Source: CAD feature listing. Evaluate the final solid. Frame: model axes, mm. Face numbers are marked on the shaded views. Round coordinates to 2 decimals unless told otherwise and drop trailing zeros. Write each loop counter-clockwise with the first axis right and the second up, starting at its lowest first coordinate (ties: lowest second). Pieces come first, ordered by that corner, then holes. Notation, with made-up numbers: M 57,-8 L 97,-8 A24 cw 97,5 Z; hole C 50,36 d6. An arc over 180 degrees is marked long. Use a Markdown table: item, result.
```python
from build123d import *

# Parameters (mm, degrees)
BOSS_EXTRUDE1_DEPTH = 10
SKETCH2_R           = 20.5
CUT_EXTRUDE1_DEPTH  = 5
SKETCH4_R           = 5
CUT_EXTRUDE3_DEPTH  = 166.604951617
SKETCH5_R           = 5
CUT_EXTRUDE4_DEPTH  = 5


with BuildPart() as part:
    # Sketch1 → Boss-Extrude1 (new body)
    with BuildSketch(Plane(origin=(0, 0, 0), x_dir=(0, 0, -1), z_dir=(1, 0, 0))):
        Polygon((-95, 70), (-140, 70), (-140, 55), (-150, 55), (-150, 15), (-140, 15), (-140, 0), (-95, 0), (-95, 5), (-55, 5), (-55, 0), (-10, 0), (-10, 15), (0, 15), (0, 55), (-10, 55), (-10, 70), (-55, 70), (-55, 60), (-95, 60), align=None)
    extrude(amount=BOSS_EXTRUDE1_DEPTH)

    # Sketch2 → Cut-Extrude1 (cut)
    with BuildSketch(Plane(origin=(10, 0, 0), x_dir=(0, 0, -1), z_dir=(1, 0, 0))):
        with Locations((-108.52, 40)):
            Circle(SKETCH2_R)
    extrude(amount=-CUT_EXTRUDE1_DEPTH, mode=Mode.SUBTRACT)

    # Sketch4 → Cut-Extrude3 (cut, through all)
    with BuildSketch(Plane(origin=(5, 0, 0), x_dir=(0, 0, -1), z_dir=(1, 0, 0))):
        with Locations((-108.52, 40)):
            Circle(SKETCH4_R)
    extrude(amount=-CUT_EXTRUDE3_DEPTH, mode=Mode.SUBTRACT)

    # Sketch5 → Cut-Extrude4 (cut)
    with BuildSketch(Plane.ZY):
        with Locations((37.080096083, 26.674400393)):
            Circle(SKETCH5_R)
        with Locations((72.52, 33)):
            Circle(SKETCH5_R)
    extrude(amount=-CUT_EXTRUDE4_DEPTH, mode=Mode.SUBTRACT)


solid = part.part
```
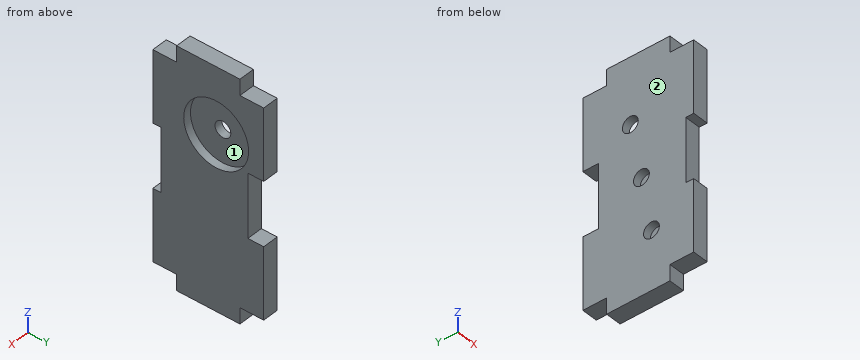
Q1. Section D-D on y = 40. Return loops of the section in (x, z).
Results are:
| item | result |
|---|---|
| outline | M 0,0 L 10,0 L 10,88.02 L 5,88.02 L 5,103.52 L 0,103.52 Z; M 0,113.52 L 5,113.52 L 5,129.02 L 10,129.02 L 10,150 L 0,150 Z |
Q2. Section A-A on z = 108.52. Return loops of the section in (x, y).
Results are:
| item | result |
|---|---|
| outline | M 0,0 L 10,0 L 10,19.5 L 5,19.5 L 5,35 L 0,35 Z; M 0,45 L 5,45 L 5,60.5 L 10,60.5 L 10,70 L 0,70 Z |
Q3. Line query: L1, parallel to Z at x = 4, y = 65.5; L2, parallel to Z at x = 2, y = 32.5; L3, parallel to Z at x = 2.5, y = 29. Output: solid intervals per line, ascending.
Results are:
| item | result |
|---|---|
| L1 | 10 to 55, 95 to 140 |
| L2 | 0 to 67.55, 77.49 to 150 |
| L3 | 0 to 32.65, 41.51 to 69.52, 75.52 to 150 |
Q4. Mould query, pull axis Y, two halves, no side actions, for the marked faces 1 and 2. Classes: +Y half, -Y half, draft (parallel to the pull), parting line (faces both ways), or undercut.
Results are:
| item | result |
|---|---|
| face 1 | undercut |
| face 2 | draft |
Q5. Section C-C on x = 6.75. Return loops of the section in (y, z), plus the area to 3 significant figures.
Results are:
| item | result |
|---|---|
| outline | M 0,10 L 15,10 L 15,0 L 55,0 L 55,10 L 70,10 L 70,55 L 60,55 L 60,95 L 70,95 L 70,140 L 55,140 L 55,150 L 15,150 L 15,140 L 0,140 L 0,95 L 5,95 L 5,55 L 0,55 Z; hole C 40,108.52 d41 |
| area | 7,980 mm^2 |
Q6. Section B-B on y = 66.5. Return loops of the section in (x, z).
Results are:
| item | result |
|---|---|
| outline | M 0,10 L 10,10 L 10,55 L 0,55 Z; M 0,95 L 10,95 L 10,140 L 0,140 Z |
Q7. First-contact query: pin 1 Ø3 at (x, y) = (6, 10) entering from -Z; pin 2 Ø5 at (x, z) = (6.5, 84.5) entering from -Y; pin 3 Ø6 at (y, z) = (40, 108.52) entering from -X; pin 4 Ø3 at (y, z) = (30.5, 73) entering from -X. Flat tips, straight axial feed; report the tip coordinate or a pass-through.
Results are:
| item | result |
|---|---|
| pin 1 | z = 10 |
| pin 2 | y = 5 |
| pin 3 | through |
| pin 4 | x = 5 |
